Input: part model. Units: mm. Frame: model coordinates. Coordinates: 2 decimals unless noted, no trailing zeros. Write each loop counter-clockwise with the first axis right and the second up, starting at its lowest first coordinate (ties: lowest second). Pieces come first, ordered by that corner, then holes. Notation, with made-up numbers: M 54.5,8 L 109.5,8 A34 cw 109.5,39 Z; hole C -18,4 d3. An arc over 180 degrees is marked long. Use one line per item in the form item = value.
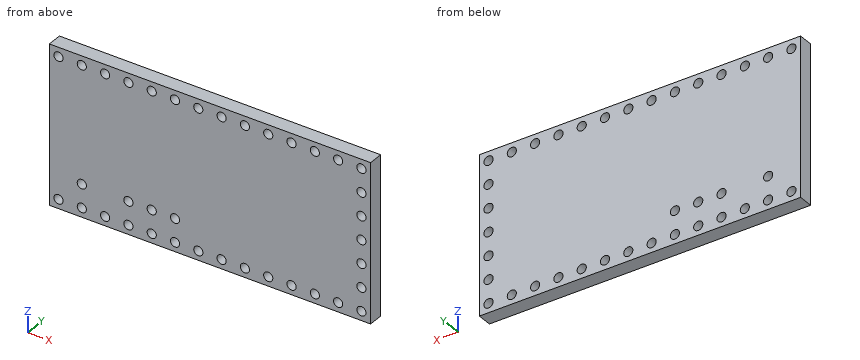
from build123d import *

# Parameters (mm, degrees)
SKETCH1_W           = 35.02
SKETCH1_H           = 17.24
BOSS_EXTRUDE1_DEPTH = 1.6
SKETCH2_R           = 0.5
CUT_EXTRUDE1_DEPTH  = 1.6
LPATTERN1_COUNT     = 14
LPATTERN1_PITCH     = 2.54
LPATTERN1_COL_COUNT = 7
LPATTERN1_COL_PITCH = 2.54
LPATTERN2_OUTLINE_R = 0.5
LPATTERN2_DEPTH     = 1.6
SKETCH3_R           = 0.5
CUT_EXTRUDE2_DEPTH  = 1.6


# Read off the part's stored shape, not the designer's step: LPattern2
with BuildPart() as part:
    # Sketch1 → Boss-Extrude1 (new body)
    with BuildSketch(Plane(origin=(0, 0, 0), x_dir=(1, 0, 0), z_dir=(0, 1, 0))):
        Rectangle(SKETCH1_W, SKETCH1_H)
    extrude(amount=BOSS_EXTRUDE1_DEPTH)

    # Sketch2 → Cut-Extrude1 (cut)
    with BuildSketch(Plane(origin=(0, 1.6, 0), x_dir=(1, 0, 0), z_dir=(0, 1, 0))):
        with Locations(Location((16.51, -7.62, 0), (0, 0, 270))):
            Circle(SKETCH2_R)
    cut_extrude1 = extrude(amount=-CUT_EXTRUDE1_DEPTH, mode=Mode.SUBTRACT)

    # LPattern1: Cut-Extrude1 ×14
    with Locations(*[(-i * LPATTERN1_PITCH, 0, 0) for i in range(1, LPATTERN1_COUNT)]):
        add(cut_extrude1, mode=Mode.SUBTRACT)

    # LPattern1 col: Cut-Extrude1 ×7
    with Locations(*[(0, 0, -i * LPATTERN1_COL_PITCH) for i in range(1, LPATTERN1_COL_COUNT)]):
        add(cut_extrude1, mode=Mode.SUBTRACT)

    # LPattern2 outline → LPattern2 (cut)
    with BuildSketch(Plane(origin=(0, 0, 0), x_dir=(1, 0, 0), z_dir=(0, 1, 0))):
        with Locations((-16.51, 7.62)):
            Circle(LPATTERN2_OUTLINE_R)
        with Locations((-13.97, 7.62)):
            Circle(LPATTERN2_OUTLINE_R)
        with Locations((-11.43, 7.62)):
            Circle(LPATTERN2_OUTLINE_R)
        with Locations((-8.89, 7.62)):
            Circle(LPATTERN2_OUTLINE_R)
        with Locations((-6.35, 7.62)):
            Circle(LPATTERN2_OUTLINE_R)
        with Locations((-3.81, 7.62)):
            Circle(LPATTERN2_OUTLINE_R)
        with Locations((-1.27, 7.62)):
            Circle(LPATTERN2_OUTLINE_R)
        with Locations((1.27, 7.62)):
            Circle(LPATTERN2_OUTLINE_R)
        with Locations((3.81, 7.62)):
            Circle(LPATTERN2_OUTLINE_R)
        with Locations((6.35, 7.62)):
            Circle(LPATTERN2_OUTLINE_R)
        with Locations((8.89, 7.62)):
            Circle(LPATTERN2_OUTLINE_R)
        with Locations((11.43, 7.62)):
            Circle(LPATTERN2_OUTLINE_R)
        with Locations((13.97, 7.62)):
            Circle(LPATTERN2_OUTLINE_R)
    extrude(amount=LPATTERN2_DEPTH, mode=Mode.SUBTRACT)

    # Sketch3 → Cut-Extrude2 (cut)
    with BuildSketch(Plane(origin=(0, 1.6, 0), x_dir=(1, 0, 0), z_dir=(0, 1, 0))):
        with Locations(Location((-13.97, 5.08, 0), (0, 0, 270))):
            Circle(SKETCH3_R)
        with Locations(Location((-8.89, 5.08, 0), (0, 0, 270))):
            Circle(SKETCH3_R)
        with Locations(Location((-6.35, 5.08, 0), (0, 0, 270))):
            Circle(SKETCH3_R)
        with Locations(Location((-3.81, 5.08, 0), (0, 0, 270))):
            Circle(SKETCH3_R)
    extrude(amount=-CUT_EXTRUDE2_DEPTH, mode=Mode.SUBTRACT)


solid = part.part
(1) Section query A-A on x = -11.43. Return the cut outline in (y, z).
Computed:
outline = M 0,-8.62 L 1.6,-8.62 L 1.6,-8.12 L 0,-8.12 Z; M 0,-7.12 L 1.6,-7.12 L 1.6,7.12 L 0,7.12 Z; M 0,8.12 L 1.6,8.12 L 1.6,8.62 L 0,8.62 Z
(2) Section query C-C on z = 2.54. Return the cut outline in (x, y).
Computed:
outline = M -17.51,0 L 16.01,0 L 16.01,1.6 L -17.51,1.6 Z; M 17.01,0 L 17.51,0 L 17.51,1.6 L 17.01,1.6 Z
(3) Section query B-B on z = -5.08. Return the cut outline in (x, y), plus the area to 3 significant figures.
Computed:
outline = M -17.51,0 L -14.47,0 L -14.47,1.6 L -17.51,1.6 Z; M -13.47,0 L -9.39,0 L -9.39,1.6 L -13.47,1.6 Z; M -8.39,0 L -6.85,0 L -6.85,1.6 L -8.39,1.6 Z; M -5.85,0 L -4.31,0 L -4.31,1.6 L -5.85,1.6 Z; M -3.31,0 L 16.01,0 L 16.01,1.6 L -3.31,1.6 Z; M 17.01,0 L 17.51,0 L 17.51,1.6 L 17.01,1.6 Z
area = 48.0 mm^2
(4) Line query: probe 1 along X at (y, z) = (0.9, -5.08); probe 2 along Z at (x, y) = (1.5, 0.3); probe 3 along Z at (x, y) = (-9, 1). Output: solid intervals per line, ascending.
Computed:
probe_1 = -17.51 to -14.47, -13.47 to -9.39, -8.39 to -6.85, -5.85 to -4.31, -3.31 to 16.01, 17.01 to 17.51
probe_2 = -8.62 to -8.06, -7.18 to 7.18, 8.06 to 8.62
probe_3 = -8.62 to -8.11, -7.13 to -5.57, -4.59 to 7.13, 8.11 to 8.62
(5) Section query D-D on y = 1.35. State how many separate pieces and enclosed holes the cut face has, plus the area to 3 significant figures.
Computed:
separate_pieces = 1
enclosed_holes = 37
area = 575 mm^2
